from build123d import *

# Parameters (mm, degrees)
F0_W     = 19.05
F0_H     = 76.2
F1_DEPTH = 19.05
F2_W     = 12.7
F2_H     = 12.7
F3_DEPTH = 76.201
F4_R     = 1.5875
F5_DEPTH = 3.175


with BuildPart() as f1:
    # F0 (on Front) → F1 (new body)
    with BuildSketch(Plane.XZ):
        with Locations((-85.803381, 38.1)):
            Rectangle(F0_W, F0_H)
    extrude(amount=F1_DEPTH)

    # F2 (on face) → F3 (cut, through all)
    with BuildSketch(Plane.XY.offset(76.2)):
        with Locations((-85.803381, -9.525)):
            Rectangle(F2_W, F2_H)
    extrude(amount=-F3_DEPTH, mode=Mode.SUBTRACT)

    # F4 (on face) → F5 (cut)
    with BuildSketch(Plane(origin=(-95.328381, 0, 0), x_dir=(0, -1, 0), z_dir=(-1, 0, 0))):
        with Locations((9.525, 57.15)):
            Circle(F4_R)
        with Locations((9.525, 19.05)):
            Circle(F4_R)
    extrude(amount=-F5_DEPTH, mode=Mode.SUBTRACT)


solid = f1.part
Could you check a few things on this model? Use its own coordinates, in mm. A direction names the side the tool comes from. Round coordinates to 2 decimals unless told otherwise and drop trailing zeros. Loops run counter-clockwise (first coordinate to the right, second up) from the corner with the lowest first, then second, coordinate; pieces in that order, holes last. Notation, with made-up numbers: (-32, 78.5) - (-10, 78.5) arc R28 ccw to (-10, 114.5) - close; hole circle Ø6 at (-40, -35.75). An arc over 180 degrees is marked (long way). Write item = value, one per line.
1) I'm going to push a flat-ended pin straight in: P1, Ø6, axis at x = -83.5, y = -10, coming from the -Z side. Where does the tip first touch, or does it pass through?
Computed:
P1 = through
2) On a 3-axis mill with a long thin cutter (end or side, diameter ignored), from which of +Z, -Z, +X, -X, +Y, -Y can I reach the whole of each face in a straight line? I mean faces 5 (the flat face through (-86, -3, 0)), 6 (the cylindrical face through (-93.76, -7.94, 19.12)), 7 (the flat face through (-92.153, -10, 39)). Say none if no direction works.
Computed:
face_5 = -Z, +X, -X, +Y, -Y
face_6 = -X
face_7 = +Z, -Z
3) I need wall thicknesses on line 1 along X through (y, z) = (-10.5, 27); line 2 along Y through (x, z) = (-86.5, 38.5) (3 decimals). Which ranges of each line are inside material? Lowest first, please. Write a range as from..to.
Computed:
line_1 = -95.33..-92.15, -79.45..-76.28
line_2 = -19.05..-15.875, -3.175..0
4) Imagine slicing it at A-A (y = -6.25). Please give me the cut outline in (x, z).
Computed:
outline = (-95.33, 0) - (-92.15, 0) - (-92.15, 76.2) - (-95.33, 76.2) - close; (-79.45, 0) - (-76.28, 0) - (-76.28, 76.2) - (-79.45, 76.2) - close
5) Imagine slicing it at C-C (z = 10.5). Please give me the cut outline in (x, y) (3 decimals), and give its area (3 significant figures).
Computed:
outline = (-95.328, -19.05) - (-76.278, -19.05) - (-76.278, 0) - (-95.328, 0) - close; hole (-92.153, -15.875) - (-79.453, -15.875) - (-79.453, -3.175) - (-92.153, -3.175) - close
area = 202 mm2
6) Imagine slicing it at B-B (x = -83.5). Please give me the cut outline in (y, z) (3 decimals).
Computed:
outline = (-19.05, 0) - (-15.875, 0) - (-15.875, 76.2) - (-19.05, 76.2) - close; (-3.175, 0) - (0, 0) - (0, 76.2) - (-3.175, 76.2) - close
7) If we mould it in two halves opening along Y, with no side actions, what happens to faces 1 (the flat face through (-86, -3.175, 39)), 2 (the flat face through (-86, -3, 76.2)), 3 (the cylindrical face through (-93.76, -9.18, 55.6)), 4 (the flat face through (-86, 0, 39))? For each: pulls with the +Y half, pulls with the -Y half, needs draft (parallel to the pull), parting line crosses it, or undercut.
Computed:
face_1 = undercut
face_2 = needs draft
face_3 = undercut
face_4 = pulls with the +Y half
